Input: part model. Units: mm. Frame: model coordinates. Round coordinates to 2 decimals unless told otherwise and drop trailing zeros. Write each loop counter-clockwise with the first axis right and the second up, starting at its lowest first coordinate (ties: lowest second). Pieces come first, ordered by that corner, then holes. Notation, with made-up numbers: (-19, 17.5) -> (-8, 17.5) arc R12 ccw to (-8, 38.5) -> close; hole circle Ø3 at (-4.75, 54.25). An arc over 180 degrees is marked (long way). Write item = value, one per line. Start each with the question number.
```python
from build123d import *

# Parameters (mm, degrees)
IMPORTED_START                = -3
IMPORTED_BODY_4_1_OUTLINE_W   = 30
IMPORTED_BODY_4_1_OUTLINE_H   = 2.8
IMPORTED_BODY_4_1_OUTLINE_H_2 = 14
IMPORTED_BODY_4_1_DEPTH       = 3
SKETCH_1_R                    = 3.5
SKETCH_1_R_2                  = 6
CUT_EXTRUDE_1_DEPTH           = 3


# Read off the part's stored shape, not the designer's step: 基体零件-零件4-1
with BuildPart() as part:
    # 基体零件-零件4-1 outline → 基体零件-零件4-1 (new body)
    with BuildSketch(Plane.XY.offset(IMPORTED_START)):
        Polygon((0, 0), (0, -3), (10, -3), (10, 0), (40, 0), (40, -3), (60, -3), (60, 0), (90, 0), (90, -3), (110, -3), (110, 0), (140, 0), (140, -3), (160, -3), (160, 0), (190, 0), (190, -3), (210, -3), (210, 0), (240, 0), (240, -3), (260, -3), (260, 0), (290, 0), (290, -3), (300.000000004, -3), (300.000000004, 0), (303.000000004, 0), (303.000000004, 30), (300.000000004, 30), (300.000000004, 104), (290, 104), (290, 100.999999998), (260, 100.999999998), (260, 103.999999998), (240, 103.999999998), (240, 100.999999998), (210, 100.999999998), (210, 103.999999998), (190, 103.999999998), (190, 100.999999998), (160, 100.999999998), (160, 103.999999998), (140, 103.999999998), (140, 100.999999998), (110, 100.999999998), (110, 103.999999998), (90, 103.999999998), (90, 100.999999998), (60, 100.999999998), (60, 103.999999998), (40, 103.999999998), (40, 100.999999998), (10, 100.999999998), (10, 103.999999998), (0, 103.999999998), (0, 81.999999998), (-3, 81.999999998), (-3, 51.999999998), (0, 51.999999998), (0, 30), (-3, 30), (-3, 0), align=None)
        with Locations((25, 62.6)):
            Rectangle(IMPORTED_BODY_4_1_OUTLINE_W, IMPORTED_BODY_4_1_OUTLINE_H, mode=Mode.SUBTRACT)
        with Locations((75, 62.6)):
            Rectangle(IMPORTED_BODY_4_1_OUTLINE_W, IMPORTED_BODY_4_1_OUTLINE_H, mode=Mode.SUBTRACT)
        with Locations((125, 57)):
            Rectangle(IMPORTED_BODY_4_1_OUTLINE_W, IMPORTED_BODY_4_1_OUTLINE_H_2, mode=Mode.SUBTRACT)
    extrude(amount=IMPORTED_BODY_4_1_DEPTH)

    # 草图1 → 切除-拉伸1 (cut)
    with BuildSketch(Plane(origin=(0, 0, -3), x_dir=(-1, 0, 0), z_dir=(0, 0, -1))):
        with Locations(Location((-147.5, 10, 0), (0, 0, 180))):
            Circle(SKETCH_1_R)
        with Locations(Location((-147.5, 45, 0), (0, 0, 180))):
            Circle(SKETCH_1_R)
        with Locations(Location((-155.5, 27.5, 0), (0, 0, 180))):
            Circle(SKETCH_1_R_2)
        with Locations((-25, 85.991178075)):
            Circle(SKETCH_1_R_2)
        with BuildLine():
            Line((-125, 31), (-98.5, 31))
            Line((-98.5, 31), (-98.5, 64.5))
            ThreePointArc((-98.5, 64.5), (-95, 68), (-91.5, 64.5))
            Line((-91.5, 64.5), (-91.5, 4))
            ThreePointArc((-91.5, 4), (-95, 0.5), (-98.5, 4))
            Line((-98.5, 4), (-98.5, 24))
            Line((-98.5, 24), (-125, 24))
            ThreePointArc((-125, 24), (-128.5, 27.5), (-125, 31))
        make_face()
    extrude(amount=-CUT_EXTRUDE_1_DEPTH, mode=Mode.SUBTRACT)


solid = part.part
```
1. Section A-A (x = 25). Output: boundary loops of the cut face in (y, z).
2. Mould query, pull axis X, two halves, no side actions, for faces 1 (the flat face through (148, 51, -3)), 2 (the cylindrical face through (26.301, 80.134, -1.521)). Classes: pulls with the +X half, pulls with the -X half, needs draft (parallel to the pull), parting line crosses it, or undercut.
3. Section C-C (x = 215). Output: boundary loops of the cut face in (y, z).
4. Section D-D (z = -1.45). State how many separate pieces and enclosed holes the cut face has, then the cut area to 3 significant figures.
5. Section B-B (y = 58). Output: boundary loops of the cut face in (x, z).
6. Line query: line 1 along Y through (x, z) = (120.5, -2.05); line 2 along X through (y, z) = (54.5, -0.95); line 3 along Y through (x, z) = (147.5, -1.05). Output: solid intervals per line, ascending.
7. Pin query (flat end, axial travel): P1, Ø0.9, axis at y = 42.5, z = -2, coming from the -X side; P2, Ø1.5, axis at x = 19.5, z = -1, coming from the -Y side; P3, Ø1.5, axis at y = -2, z = -1, coming from the +X side. Return the tip coordinate at first contact, or that it passes through.
Check sheet entries:
q1.outline = (0, -3) -> (61.2, -3) -> (61.2, 0) -> (0, 0) -> close; (64, -3) -> (79.99, -3) -> (79.99, 0) -> (64, 0) -> close; (91.99, -3) -> (101, -3) -> (101, 0) -> (91.99, 0) -> close
q2.face_1 = needs draft
q2.face_2 = undercut
q3.outline = (0, -3) -> (101, -3) -> (101, 0) -> (0, 0) -> close
q4.separate_pieces = 1
q4.enclosed_holes = 8
q4.area = 29,700 mm2
q5.outline = (-3, -3) -> (91.5, -3) -> (91.5, 0) -> (-3, 0) -> close; (98.5, -3) -> (110, -3) -> (110, 0) -> (98.5, 0) -> close; (140, -3) -> (300, -3) -> (300, 0) -> (140, 0) -> close
q6.line_1 = 0 to 24, 31 to 50, 64 to 101
q6.line_2 = -3 to 91.5, 98.5 to 110, 140 to 300
q6.line_3 = -3 to 6.5, 13.5 to 41.5, 48.5 to 104
q7.P1 = 0
q7.P2 = 0
q7.P3 = 300
